Autodesk Inventor part; units mm, degrees
ref_plane "YZ Plane" through (0, 0, 0) normal (1, 0, 0) x (0, 1, 0)
ref_plane "XZ Plane" through (0, 0, 0) normal (0, 1, 0) x (-1, 0, 0)
ref_plane "XY Plane" through (0, 0, 0) normal (0, 0, 1) x (1, 0, 0)
sketch "Block1" plane through (0, 0, 0) normal (0, 0, 1) x (1, 0, 0)
  arc A0 (4.4042, -0.6007) -> (-4.4042, -0.6007) centre (0, 0) ccw
  arc A1 (-2.5167, -14.4402) -> (2.5167, -14.4402) centre (0, -14.097) ccw
  line L0 (-2.5167, -14.4402) -> (-4.4042, -0.6007)
  line L1 (4.4042, -0.6007) -> (2.5167, -14.4402)
  line L2 (-7.5501, -1.0297) -> (-5.6626, -14.8693)
  arc A2 (-5.6626, -14.8693) -> (5.6626, -14.8693) centre (0, -14.097) ccw
  line L3 (5.6626, -14.8693) -> (7.5501, -1.0297)
  arc A3 (7.5501, -1.0297) -> (-7.5501, -1.0297) centre (0, 0) ccw
  line L4 (-4.9018, -0.6685) -> (-3.0142, -14.5081)
  arc A4 (-3.0142, -14.5081) -> (3.0142, -14.5081) centre (0, -14.097) ccw
  line L5 (3.0142, -14.5081) -> (4.9018, -0.6685)
  arc A5 (4.9018, -0.6685) -> (-4.9018, -0.6685) centre (0, 0) ccw
  point P0 (0, -7.4025)
  dimension "d127" = 8.89
  dimension "d131" = 5.08
  dimension "d140" = 3.175
sketch "Sketch10" plane through (0, 0, 0) normal (0, 1, 0) x (-1, 0, 0)
  circle A0 centre (0, 0) radius 8.636
  line L0 (0, -14.097) -> (0, 0)
  arc A1 (-4.826, 10.0803) -> (-4.826, -10.0803) centre (0, 0) ccw
  circle A2 centre (0, 0) radius 11.176
  circle A3 centre (0, 0) radius 12.446
  line L1 (-12.7635, 23.7871) -> (12.7635, 23.7871)
  line L2 (0, 23.7871) -> (0, -23.7871)
  line L3 (-12.7635, -23.7871) -> (12.7635, -23.7871)
  line L4 (-2.032, 23.7871) -> (-2.032, -23.7871)
  line L5 (2.032, 23.7871) -> (2.032, -23.7871)
  line L6 (0, 11.176) -> (0, -22.606)
  line L7 (0, 11.176) -> (0, -22.606)
  arc A4 (4.4042, -0.6007) -> (-4.4042, -0.6007) centre (0, 0) ccw
  arc A5 (-2.5167, -14.4402) -> (2.5167, -14.4402) centre (0, -14.097) ccw
  line L8 (-2.5167, -14.4402) -> (-4.4042, -0.6007)
  line L9 (4.4042, -0.6007) -> (2.5167, -14.4402)
  line L10 (-7.5501, -1.0297) -> (-5.6626, -14.8693)
  arc A6 (-5.6626, -14.8693) -> (5.6626, -14.8693) centre (0, -14.097) ccw
  line L11 (5.6626, -14.8693) -> (7.5501, -1.0297)
  arc A7 (7.5501, -1.0297) -> (-7.5501, -1.0297) centre (0, 0) ccw
  line L12 (-4.9018, -0.6685) -> (-3.0142, -14.5081)
  arc A8 (-3.0142, -14.5081) -> (3.0142, -14.5081) centre (0, -14.097) ccw
  line L13 (3.0142, -14.5081) -> (4.9018, -0.6685)
  arc A9 (4.9018, -0.6685) -> (-4.9018, -0.6685) centre (0, 0) ccw
  point P0 (2.032, -10.9897)
  point P1 (2.032, -12.279)
  point P2 (-2.032, -12.279)
  point P3 (-2.032, -10.9897)
  point P4 (-2.032, 10.9897)
  point P5 (2.032, 10.9897)
  point P6 (-6.1771, -11.0965)
  point P7 (6.1771, -11.0965)
  point P8 (6.4453, -9.1302)
  point P9 (7.0009, -5.0565)
  point P10 (2.032, 8.3935)
  point P11 (-2.032, 8.3935)
  point P12 (-7.0009, -5.0565)
  point P13 (-6.4453, -9.1302)
  point P14 (6.1771, -11.0965)
  point P15 (-6.1771, -11.0965)
  point P16 (2.032, 7.3441)
  point P17 (-7.0009, -5.0565)
  point P18 (7.0009, -5.0565)
  point P19 (6.4453, -9.1302)
  point P20 (2.032, -19.4386)
  point P21 (-6.4453, -9.1302)
  point P22 (2.032, -8.3935)
  point P23 (-2.032, 7.3441)
  point P24 (-2.032, -19.4386)
  point P25 (-2.032, -8.3935)
  point P26 (6.2203, -10.7801)
  point P27 (-6.2203, -10.7801)
  point P28 (2.032, 7.3441)
  point P29 (-7.0009, -5.0565)
  point P30 (7.0009, -5.0565)
  point P31 (6.4453, -9.1302)
  point P32 (2.032, -19.4386)
  point P33 (-6.4453, -9.1302)
  point P34 (-2.032, 7.3441)
  point P35 (-2.032, -19.4386)
  point P36 (-6.4453, -9.1302)
  dimension "d149" = 24.892
  dimension "d148" = 2.032
  dimension "d147" = 2.032
  dimension "d146" = 33.782
  dimension "d159" = 33.782
extrude "Extrusion21" add sketch "Sketch10" against normal blind 17.145 contours L5 A3 L11 A2 | A2 L2 A3 L5 | L11 A3 L13 A2 | A2 L4 A3 L2 | L13 A3 L9 A2 | A2 A1 L10 A3 L4 | L9 A3 L5 A2 | A1 A2 L12 A3 L10 | A2 L8 A3 L12 | A2 L4 A3 L8
extrude "Extrusion22" add sketch "Sketch10" against normal blind 8.128 contours A0 L11 A7 L5 | A0 L5 A2 L11 | L11 A2 L13 A0 | A0 L13 A9 L5 A7 L11 | L13 A2 L9 A0 | A0 L9 A4 L5 A9 L13 | L4 A7 L10 A0 | A0 L10 A1 A2 L4 | L9 A2 L5 A0 | A0 L5 A4 L9 | L10 A7 L4 A9 L12 A0 | A0 L12 A2 A1 L10 | L12 A9 L4 A4 L8 A0 | A0 L8 A2 L12 | L8 A4 L4 A0 | A0 L4 A2 L8
extrude "Extrusion23" add sketch "Sketch10" along normal blind 6.731 contours A0 L11 A7 L5 | L5 A7 L2 A0 | A0 L2 A2 L5 | L11 A2 L13 A0 | A0 L13 A9 L5 A7 L11 | L2 A7 L4 A0 | A0 L4 A2 L2 | L5 A3 L11 A2 | A2 L2 A3 L5 | L5 A9 L2 A7 | L13 A2 L9 A0 | A0 L9 A4 L5 A9 L13 | L11 A3 L13 A2 | L4 A7 L10 A0 | A2 L4 A3 L2 | L2 A9 L4 A7 | L5 A4 L2 A9 | L13 A3 L9 A2 | L11 A6 L5 A8 L13 A3 | L10 A7 L4 A9 L12 A0 | A0 L12 A2 A1 L10 | A2 A1 L10 A3 L4 | L2 A4 L4 A9 | L13 A8 L5 A5 L9 A3 | L12 A9 L4 A4 L8 A0 | A0 L8 A2 L12 | A1 A2 L12 A3 L10 | A6 L2 A8 L5 | A2 L8 A3 L12 | A3 L12 A8 L4 A6 L10 | A8 L2 A5 L5 | A6 L4 A8 L2 | A3 L8 A5 L4 A8 L12 | A8 L4 A5 L2
extrude "Extrusion24" cut sketch "Sketch10" along normal blind 6.096 contours L13 A2 L9 A0 | A0 L9 A4 L5 A9 L13 | L5 A4 L2 A9 | L9 A2 L5 A0 | A0 L5 A4 L9 | L13 A3 L9 A2 | L2 A4 L4 A9 | L5 A0 L0 L2 A4 | L5 A2 L0 A0 | L9 A3 L5 A2 | L13 A8 L5 A5 L9 A3 | L12 A9 L4 A4 L8 A0 | A0 L8 A2 L12 | L2 L0 A0 L4 A4 | L0 A2 L4 A0 | L5 A3 L0 A2 | L9 A5 L5 A3 | L8 A4 L4 A0 | A0 L4 A2 L8 | A2 L8 A3 L12 | L0 A3 L4 A2 | L5 A5 L2 L0 A3 | A8 L2 A5 L5 | A2 L4 A3 L8 | A3 L8 A5 L4 A8 L12 | L0 L2 A5 L4 A3 | A8 L4 A5 L2 | A3 L4 A5 L8
properties part number "Servo Adapter 4"
Geometry check sheet. Reference: the model listing, model coordinates, mm. A direction names the side the tool comes from. Give positions to 0.01 mm unless a question says otherwise; leave off trailing zeros. Order: outer loops, then holes, each group sorted by start corner. A loop starts at its lowest first (then second) coordinate and runs counter-clockwise, first axis right, second up. Notation, with made-up numbers: (72, 7.5) - (78, 7.5) arc R14 cw to (78, 27.5) - close; hole circle Ø10 at (56, 9.25). An arc over 180 degrees is marked (long way). Answer as a JSON object with one key per item and string values.
(1) Cross-section at A-A (x = 0). Record the cut outline in (y, z) (3 decimals), then the cut area to 3 significant figures.
Report:
{"outline": "(-17.145, 11.176) - (0, 11.176) - (0, 4.947) - (6.096, 4.947) - (6.096, 4.445) - (6.731, 4.445) - (6.731, 12.446) - (-17.145, 12.446) - close; (0, -19.812) - (6.731, -19.812) - (6.731, -16.637) - (6.096, -16.637) - (6.096, -17.139) - (0, -17.139) - close", "area": "90.9 mm^2"}
(2) Cross-section at D-D (z = 8). Record the cut outline in (x, y) (3 decimals), then the cut area to 3 significant figures.
Report:
{"outline": "(-9.534, -17.145) - (-7.804, -17.145) - (-7.804, -8.128) - (-2.032, -8.128) - (-2.032, 0) - (2.032, 0) - (2.032, -8.128) - (7.804, -8.128) - (7.804, -17.145) - (9.534, -17.145) - (9.534, 6.731) - (7.804, 6.731) - (7.804, 0) - (3.253, 0) - (3.253, 6.731) - (-3.253, 6.731) - (-3.253, 0) - (-7.804, 0) - (-7.804, 6.731) - (-9.534, 6.731) - close", "area": "220 mm^2"}
(3) Cross-section at C-C (y = 1.25). Record the cut outline in (x, z), then the cut area to 3 significant figures.
Report:
{"outline": "(-6.22, -10.78) - (-5.66, -14.87) arc R5.72 ccw to (5.66, -14.87) - (6.22, -10.78) arc R12.45 ccw (long way) to start; hole (-7, -5.06) arc R8.64 cw to (-2.03, 8.39) - (-2.03, 10.99) arc R11.18 ccw to (-6.45, -9.13) - close; hole (-4.9, -0.67) - (-3.01, -14.51) arc R3.04 ccw to (3.01, -14.51) - (4.9, -0.67) arc R4.95 ccw (long way) to start; hole (2.03, 8.39) arc R8.64 cw to (7, -5.06) - (6.45, -9.13) arc R11.18 ccw to (4.83, 10.08) arc R11.18 ccw to (2.03, 10.99) - close", "area": "287 mm^2"}
(4) Depth check by flat-ended pin: pin 1 Ø2 at (x, y) = (1.5, -5.5) entering from +Z; pin 2 Ø4.5 at (x, z) = (0.5, 8) entering from -Y; pin 3 Ø1.5 at (x, z) = (3.5, -1) entering from +Y. Enter the tip coordinate at first touch or a pass-through.
Report:
{"pin 1": "z = 12.44", "pin 2": "y = -8.13", "pin 3": "y = 0"}
(5) Cross-section at B-B (z = 0). Record the cut outline in (x, y) (3 decimals), then the cut area to 3 significant figures.
Report:
{"outline": "(-12.446, -17.145) - (-11.176, -17.145) - (-11.176, -8.128) - (-2.032, -8.128) - (-2.032, 0) - (-4.947, 0) - (-4.947, 6.096) - (-4.445, 6.096) - (-4.445, 6.731) - (-8.636, 6.731) - (-8.636, 0) - (-11.176, 0) - (-11.176, 6.731) - (-12.446, 6.731) - close; (2.032, -8.128) - (11.176, -8.128) - (11.176, -17.145) - (12.446, -17.145) - (12.446, 6.731) - (11.176, 6.731) - (11.176, 0) - (8.636, 0) - (8.636, 6.731) - (4.445, 6.731) - (4.445, 6.096) - (4.947, 6.096) - (4.947, 0) - (2.032, 0) - close", "area": "260 mm^2"}
(6) Draft check along Z on faces 6 (the flat face through (4, 6.096, -6)), 7 (the cylindrical face through (-0.519, -5.04, 12.435)), 8 (the flat face through (-1.3, 0, -17.2)). Enter one of: released by +Z, released by -Z, zero draft, split by the parting line, or undercut.
Report:
{"face 6": "undercut", "face 7": "split by the parting line", "face 8": "zero draft"}
(7) Tool access check on faces 1 (the flat face through (-2.032, -3, 0)), 2 (the flat face through (6, 6.731, 0)), 3 (the flat face through (6, -8.128, 0)), 4 (the flat face through (3.97, 3.01, -7.49)), 5 (the cylindrical face through (-8.06, 3.32, 3.1)). Record the directions out of +Z, -Z, +X, -X, +Y, -Y that give a thin tool (end or side, any length) a straight path to the whole face; none if there is none.
Report:
{"face 1": "-Z, -Y", "face 2": "+Z, -Z, +X, -X, +Y", "face 3": "-Y", "face 4": "none", "face 5": "+Y"}
(8) Material ranges on line 1 (X direction, y = 6.55, z = 0); line 2 (X direction, y = -5.75, z = 0); line 3 (Z direction, x = 0, y = 6.3), recorded low to high.
Report:
{"line 1": "-12.45 to -11.18, -8.64 to -4.44, 4.44 to 8.64, 11.18 to 12.45", "line 2": "-12.45 to -2.03, 2.03 to 12.45", "line 3": "-19.81 to -16.64, 4.44 to 12.45"}
